Geometry: final body of the model. Coordinates: model frame, mm. Face numbers are marked on the shaded views. Round coordinates to 2 decimals unless told otherwise and drop trailing zeros. Order: outer loops, then holes, each group sorted by start corner. A loop starts at its lowest first (then second) coordinate and runs counter-clockwise, first axis right, second up. Notation, with made-up numbers: M -37,-30 L 12,-30 A31 cw 12,-1 Z; hole C -3.75,35.25 d8. An arc over 180 degrees is marked long. Return JSON: item names as keys, results as strings. Group by question number.
Q1. Contact query for flat-ended pins moving along their axis: pin 1 (8 mm diameter, centred on x = -11.14, z = 11.14, fed in from +Y); pin 2 (3 mm diameter, centred on y = -12, z = 13.5, fed in from +X); pin 3 (8 mm diameter, centred on x = -19.5, y = -12.5, fed in from +Z). Output: stop coordinate, or through.
Q2. Cut plane B-B on z = 0. Output: boundary loops of the cut face in (x, y), and give its area (3 significant figures).
Q3. Ray query, probe 1 along X at (y, z) = (-6, -15); probe 2 along Z at (x, y) = (-8, -4.5); probe 3 along Z at (x, y) = (-1, -10). Return the intervals inside material, ascending.
Q4. Cut plane A-A on x = 0. Output: boundary loops of the cut face in (y, z).
Q5. Cut plane D-D on z = 31.5. Output: boundary loops of the cut face in (x, y), and give its area (3 significant figures).
Q6. Mould query, pull axis X, two halves, no side actions, for the marked faces 1, 2 and 3. Classes: released by +X, released by -X, zero draft, split by the parting line, or undercut.
Q7. Cut plane C-C on x = -31.5. Output: boundary loops of the cut face in (y, z).
Autodesk Inventor part; units mm, degrees
ref_plane "YZ Plane" through (0, 0, 0) normal (1, 0, 0) x (0, 1, 0)
ref_plane "XZ Plane" through (0, 0, 0) normal (0, 1, 0) x (-1, 0, 0)
ref_plane "XY Plane" through (0, 0, 0) normal (0, 0, 1) x (1, 0, 0)
sketch "Sketch1" plane through (0, 0, 0) normal (0, 1, 0) x (-1, 0, 0)
  circle A0 centre (0, 0) radius 40
  circle A1 centre (0, 0) radius 21
  point P0 (11.1369, 11.1369)
  point P1 (-11.1369, 11.1369)
  point P2 (-11.1369, -11.1369)
  point P3 (11.1369, -11.1369)
  dimension "d0" = 80
  dimension "d2" = 15.75
  dimension "d5" = 360
  dimension "d16" = 42
extrude "Extrusion1" add sketch "Sketch1" against normal blind 15 contours A0 | A1
hole "Hole1" at (-11.1369, 0, 11.1369) at (11.1369, 0, 11.1369) at (11.1369, 0, -11.1369) at (-11.1369, 0, -11.1369) direction (0, -1, 0) diameter 5.5 end through all counterbore diameter 10 counterbore depth 8.5
extrude "Extrusion2" cut sketch "Sketch1" against normal blind 3.5 contours A1
sketch "Sketch2" plane through (0, -15, 0) normal (0, -1, 0) x (1, 0, 0)
  circle A0 centre (0, 0) radius 40
  circle A1 centre (0, 0) radius 20
  point P0 (31.5, 0)
  point P1 (22.2739, 22.2739)
  point P2 (0, 31.5)
  point P3 (-22.2739, 22.2739)
  point P4 (-31.5, 0)
  point P5 (-22.2739, -22.2739)
  point P6 (0, -31.5)
  point P7 (22.2739, -22.2739)
  point P8 (23.097, 9.5671)
  dimension "d25" = 31.5
  dimension "d26" = 40
  dimension "d29" = 360
  dimension "d38" = 25
hole "Hole2" at (22.2739, -15, 22.2739) at (31.5, -15, 0) at (22.2739, -15, -22.2739) at (0, -15, -31.5) at (-22.2739, -15, -22.2739) at (-31.5, -15, 0) at (-22.2739, -15, 22.2739) at (0, -15, 31.5) direction (0, 1, 0) diameter 6.6 end through all
properties part number "Plate"
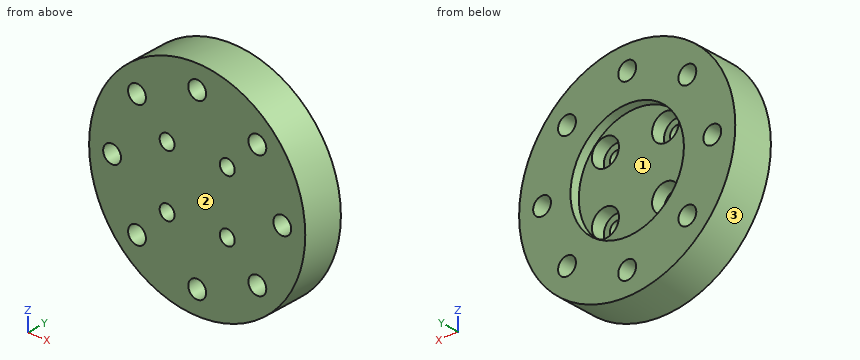
Result sheet:
{
 "1": {"pin 1": "stops at y = -8.5", "pin 2": "stops at x = 38.16", "pin 3": "stops at z = 36.87"},
 "2": {"outline": "M -40,-15 L -34.8,-15 L -34.8,0 L -40,0 Z; M -28.2,-15 L 28.2,-15 L 28.2,0 L 21,0 L 21,-3.5 L -21,-3.5 L -21,0 L -28.2,0 Z; M 34.8,-15 L 40,-15 L 40,0 L 34.8,0 Z", "area": "855 mm²"},
 "3": {"probe 1": "x = -37.08 to -14.31, -7.96 to 7.96, 14.31 to 37.08", "probe 2": "z = -39.19 to -15.03, -7.24 to 7.24, 15.03 to 39.19", "probe 3": "z = -39.99 to -34.64, -28.36 to 28.36, 34.64 to 39.99"},
 "4": {"outline": "M -15,-40 L 0,-40 L 0,-34.8 L -15,-34.8 Z; M -15,-28.2 L 0,-28.2 L 0,-21 L -3.5,-21 L -3.5,21 L 0,21 L 0,28.2 L -15,28.2 Z; M -15,34.8 L 0,34.8 L 0,40 L -15,40 Z"},
 "5": {"outline": "M -24.65,-15 L -3.3,-15 L -3.3,0 L -24.65,0 Z; M 3.3,-15 L 24.65,-15 L 24.65,0 L 3.3,0 Z", "area": "641 mm²"},
 "6": {"face 1": "undercut", "face 2": "zero draft", "face 3": "split by the parting line"},
 "7": {"outline": "M -15,-24.65 L 0,-24.65 L 0,-3.3 L -15,-3.3 Z; M -15,3.3 L 0,3.3 L 0,24.65 L -15,24.65 Z"}
}
